For this review, take the finished solid that the model builds, in its own axes (mm). Give positions to 0.01 mm unless a question says otherwise; leave off trailing zeros. Order: outer loops, then holes, each group sorted by start corner. A loop starts at its lowest first (then second) coordinate and runs counter-clockwise, first axis right, second up. Notation, with made-up numbers: (37, 11.5) - (52, 11.5) arc R25 ccw to (52, 42.5) - close; hole circle Ø9 at (71.25, 18). An arc over 180 degrees is marked (long way). Use a Markdown table: item, result. Add a question column.
1) Mouldability with a two-part tool opening along Z and no side actions: class faces 1 (the face through (-1.9, 0.08, 10.75)), 2 (the face through (0, -2, 12)), 3 (the face through (0, 0, 13)) as released by +Z, released by -Z, zero draft, split by the parting line, or undercut.
2) Wall thickness on L1, parallel to X at y = -0.1, z = 2.25; L2, parallel to Y at x = -1, z = 5; L3, parallel to X at y = -0.65, z = 1: over which ranges is each line inside the solid? List them lowest first.
3) We need section A-A on z = 3. Write out the cut boundary in (x, y).
4) Clearance check with flat-ended pins moving along their axes: P1, Ø1.5, axis at y = 1, z = 8, coming from the +X side; P2, Ø1.5, axis at x = -1, z = 3, coming from the -Y side. State where each tip first meets the part, or that it passes through.
Solid Edge part; units mm, degrees
sketch "Sketch1" plane through (0, 0, 0) normal (0, -1, 0) x (1, 0, 0)
  line L0 (0, 0) -> (2, 0)
  line L1 (2, 0) -> (2, 10.5)
  line L2 (1.9, 10.5) -> (2, 10.5)
  line L3 (1.9, 10.5) -> (1.9, 11)
  line L4 (2, 11) -> (1.9, 11)
  line L5 (2, 11) -> (2, 12.5)
  line L6 (2, 12.5) -> (1.5, 13)
  line L7 (1.5, 13) -> (0, 13)
revolve "RevolvedProtrusion1" add sketch "Sketch1" angle 360 about axis through (0, 0, 13) along (0, 0, -1)
Checked values:
| question | item | result |
|---|---|---|
| 1 | face 1 | undercut |
| 1 | face 2 | zero draft |
| 1 | face 3 | released by +Z |
| 2 | L1 | -2 to 2 |
| 2 | L2 | -1.73 to 1.73 |
| 2 | L3 | -1.89 to 1.89 |
| 3 | outline | circle Ø4 at (0, 0) |
| 4 | P1 | x = 1.98 |
| 4 | P2 | y = -1.98 |
